from build123d import *

# Parameters (mm, degrees)
SKETCH1_R           = 1.4605
BOSS_EXTRUDE1_DEPTH = 1.5875
CUT_EXTRUDE1_START  = -4.175
SKETCH2_W           = 2.921
SKETCH2_H           = 8.89
CUT_EXTRUDE1_DEPTH  = 5.175


with BuildPart() as part:
    # Sketch1 → Boss-Extrude1 (new body, symmetric)
    with BuildSketch(Plane(origin=(0, 0, 0), x_dir=(1, 0, 0), z_dir=(0, 1, 0))):
        with BuildLine():
            Line((4.284041303, -20.235333333), (9.180088507, -2.54))
            ThreePointArc((9.180088507, -2.54), (0, 9.525), (-9.180088507, -2.54))
            Line((-9.180088507, -2.54), (-4.284041303, -20.235333333))
            ThreePointArc((-4.284041303, -20.235333333), (0, -23.495), (4.284041303, -20.235333333))
        make_face()
        with Locations((0, -19.05)):
            Circle(SKETCH1_R, mode=Mode.SUBTRACT)
    extrude(amount=BOSS_EXTRUDE1_DEPTH, both=True)

    # Sketch2 → Cut-Extrude1 (cut)
    with BuildSketch(Plane(origin=(0, 1.5875, 0), x_dir=(1, 0, 0), z_dir=(0, 1, 0)).offset(CUT_EXTRUDE1_START)):
        with Locations((-3.048, -4.445)):
            Rectangle(SKETCH2_W, SKETCH2_H)
    cut_extrude1 = extrude(amount=CUT_EXTRUDE1_DEPTH, mode=Mode.SUBTRACT)

    # Mirror1: Cut-Extrude1 across plane
    add(cut_extrude1.mirror(Plane(origin=(0, 0, 0), x_dir=(0, 0, 1), z_dir=(1, 0, 0))), mode=Mode.SUBTRACT)


solid = part.part
Input: part model. Units: mm. Frame: model coordinates. A direction names the side the tool comes from. Coordinates: 2 decimals unless noted, no trailing zeros. Order: outer loops, then holes, each group sorted by start corner. A loop starts at its lowest first (then second) coordinate and runs counter-clockwise, first axis right, second up.
1. Access query for faces 5 (the cylindrical face through (-0.081, 0.022, 23.494)), 6 (the flat face through (1.588, 0, 5)). Directions: +Z, -Z, +X, -X, +Y, -Y. A direction counts if a zero-diameter tool reaches every point of the face in a straight line with its end or side. Return the directions, or none.
Checked values:
face 5: +Z, +Y, -Y
face 6: +Y, -Y
2. Cut plane C-C, the plane y = -0.5. Count the separate pieces of the cut face and the enclosed holes in it, plus the area to 3 significant figures.
Checked values:
separate pieces: 1
enclosed holes: 3
area: 391 mm2
3. Cut plane D-D, the plane z = 15.5. Return loops of the section in (x, y), plus the area to 3 significant figures.
Checked values:
outline: (-5.59, -1.59) - (5.59, -1.59) - (5.59, 1.59) - (-5.59, 1.59) - close
area: 35.5 mm2
4. Ray query, line 1 along X through (y, z) = (0, 8); line 2 along X through (y, z) = (-0.3, 6); line 3 along Z through (x, y) = (0, 0.85) (1 decimal). Return the intervals inside material, ascending.
Checked values:
line 1: x = -7.67 to -4.51, -1.59 to 1.59, 4.51 to 7.67
line 2: x = -8.22 to -4.51, -1.59 to 1.59, 4.51 to 8.22
line 3: z = -9.5 to 17.6, 20.5 to 23.5
5. Cut plane B-B, the plane z = 19.05. Return loops of the section in (x, y).
Checked values:
outline: (-4.61, -1.59) - (-1.46, -1.59) - (-1.46, 1.59) - (-4.61, 1.59) - close; (1.46, -1.59) - (4.61, -1.59) - (4.61, 1.59) - (1.46, 1.59) - close
6. Draft query along X for faces 1 (the flat face through (4.508, 0, 5)), 2 (the flat face through (0, -1.588, 3)), 3 (the flat face through (3, 0, 8.89)), 4 (the flat face through (6.7, 0, 11.5)). Return one class per face: +X half, -X half, draft (parallel to the pull), parting line (faces both ways), or undercut.
Checked values:
face 1: undercut
face 2: draft
face 3: undercut
face 4: +X half
7. Contact query for flat-ended pins moving along their axis: P1, Ø0.9, axis at x = -3, y = -0.5, coming from the +Z side; P2, Ø1, axis at y = 0.5, z = 2.5, coming from the +X side; P3, Ø1.6, axis at y = 0, z = 3.5, coming from the +X side. Output: stop coordinate, or through.
Checked values:
P1: stops at z = 22.69
P2: stops at x = 9.31
P3: stops at x = 9.14
8. Cut plane A-A, the plane x = 0. Return loops of the section in (y, z) (1 decimal), plus the area to 3 significant figures.
Checked values:
outline: (-1.6, -9.5) - (1.6, -9.5) - (1.6, 17.6) - (-1.6, 17.6) - close; (-1.6, 20.5) - (1.6, 20.5) - (1.6, 23.5) - (-1.6, 23.5) - close
area: 95.6 mm2
